Autodesk Inventor part; units mm, degrees
ref_plane "YZ Plane" through (0, 0, 0) normal (1, 0, 0) x (0, 1, 0)
ref_plane "XZ Plane" through (0, 0, 0) normal (0, 1, 0) x (-1, 0, 0)
ref_plane "XY Plane" through (0, 0, 0) normal (0, 0, 1) x (1, 0, 0)
sketch "Sketch1" plane through (0, 0, 0) normal (0, 0, 1) x (1, 0, 0)
  line L0 (0, 0) -> (30, 0)
  line L1 (30, 0) -> (30, 8)
  line L2 (30, 8) -> (0, 8)
  line L3 (0, 8) -> (0, 0)
  line L4 (14.9976, 2) -> (24.9976, 2)
  line L5 (14.9976, 2) -> (4.9976, 2)
  arc A0 (24.9976, 2) -> (4.9976, 2) centre (14.9976, -10.49) ccw
  dimension "d2" = 30
  dimension "d3" = 8
  dimension "d6" = 10
  dimension "d7" = 10
  dimension "d8" = 2
  dimension "d9" = 16
extrude "Extrusion1" add sketch "Sketch1" along normal blind 250
sketch "Sketch2" plane through (0, 8, 0) normal (0, 1, 0) x (1, 0, 0)
  line L0 (30, 0) -> (0, 0)
  line L1 (30, 0) -> (30, -250)
  circle A0 centre (15, -125) radius 5
  line L2 (30, -250) -> (0, -250)
  line L3 (10, -15) -> (10, -5)
  line L4 (10, -5) -> (20, -5)
  line L5 (20, -5) -> (20, -15)
  line L6 (20, -15) -> (10, -15)
  line L7 (10, -15) -> (20, -5) construction
  line L8 (10, -5) -> (20, -15) construction
  line L9 (0, 0) -> (0, -250)
  line L10 (10, -235) -> (10, -245)
  line L11 (10, -245) -> (20, -245)
  line L12 (20, -245) -> (20, -235)
  line L13 (20, -235) -> (10, -235)
  line L14 (10, -235) -> (20, -245) construction
  line L15 (10, -245) -> (20, -235) construction
  point P0 (15, 0)
  point P1 (30, -125)
  point P2 (15, -5)
  point P3 (15, -10)
  point P4 (15, -240)
  point P5 (15, -245)
  dimension "d13" = 10
  dimension "d14" = 120
  dimension "d16" = 0
  dimension "d17" = 125
  dimension "d19" = 5
  dimension "d20" = 10
  dimension "d21" = 10
  dimension "d22" = 5
  dimension "d23" = 10
  dimension "d24" = 5
  dimension "d25" = 5
  dimension "d26" = 10
extrude "Extrusion2" cut sketch "Sketch2" against normal up to surface (8 mm away) from surface at 0 contours A0 | L3 L4 L5 L6 | L13 L12 L11 L10
sketch "Sketch3" plane through (0, 8, 0) normal (0, 1, 0) x (1, 0, 0)
  line L0 (30, 0) -> (30, -250)
  line L1 (30, 0) -> (0, 0)
  line L2 (0, -140) -> (30, -140)
  line L3 (30, -140) -> (30, -110)
  line L4 (30, -110) -> (0, -110)
  line L5 (0, -110) -> (0, -140)
  line L6 (0, -140) -> (30, -110) construction
  line L7 (30, -140) -> (0, -110) construction
  line L8 (4.9976, 0) -> (4.9976, -250)
  point P0 (30, -125)
  point P1 (15, 0)
  point P2 (15, -125)
  dimension "d29" = 15
  dimension "d30" = 125
  dimension "d31" = 30
  dimension "d32" = 30
extrude "Extrusion3" cut sketch "Sketch3" against normal blind 5 contours L0 L2 L8 L4 | L8 L2 L5 L4
properties part number "bridge1"
The model under review builds one solid part; all positions refer to its coordinate system, in mm. A direction names the side the tool comes from. Round coordinates to 2 decimals unless told otherwise and drop trailing zeros. Write each loop counter-clockwise with the first axis right and the second up, starting at its lowest first coordinate (ties: lowest second). Pieces come first, ordered by that corner, then holes. Notation, with made-up numbers: M 43.25,-34.5 L 54.25,-34.5 A22 cw 54.25,-22.5 Z; hole C -34,-27.75 d2. An arc over 180 degrees is marked long. Answer as CSV lines item,"result". Start each with the question number.
Q1. Consider section A-A, the plane z = 94. Give the boundary of the cut face in (x, y), then the cut area to 3 significant figures.
Q2. Consider section C-C, the plane z = 125. Give the boundary of the cut face in (x, y), then the cut area to 3 significant figures.
Q3. Consider section B-B, the plane x = 15. State how many separate pieces and enclosed holes the cut face has, then the cut area to 3 significant figures.
Q4. The part is to be moulded in two halves that separate along X. For faces 1 (the face through (8, 2, 123)), 2 (the face through (0, 2, 123)), 3 (the face through (27, 3, 125)), 4 (the face through (30, 2, 123)), say which applies: +X half, -X half, draft (parallel to the pull), parting line (faces both ways), or undercut.
Q5. Tool access review of faces 5 (the face through (17.307, 1.014, 129.436)), 6 (the face through (15, 6, 140)): name each direction out of +Z, -Z, +X, -X, +Y, -Y from which nothing blocks a thin tool from reaching the whole face with its end or side.
Q6. Wall thickness on line 1 along Z through (x, y) = (15, 1.25); line 2 along Z through (x, y) = (18.5, 7.5); line 3 along X through (y, z) = (0.65, 125): over which ranges is each line inside the solid? List them lowest first.
Result set:
1,outline,"M 0,0 L 30,0 L 30,8 L 0,8 Z; hole M 5,2 L 25,2 A16 ccw Z"
1,area,"192 mm²"
2,outline,"M 0,0 L 10,0 L 10,2 L 5,2 A16 cw 6.39,3 L 0,3 Z; M 20,0 L 30,0 L 30,3 L 23.6,3 A16 cw 25,2 L 20,2 Z"
2,area,"51.3 mm²"
3,separate pieces,"8"
3,enclosed holes,"0"
3,area,"938 mm²"
4,face 1,"undercut"
4,face 2,"-X half"
4,face 3,"draft"
4,face 4,"+X half"
5,face 5,"+Y, -Y"
5,face 6,"+X, -X, +Y"
6,line 1,"z = 0 to 5, 15 to 120, 130 to 235, 245 to 250"
6,line 2,"z = 0 to 5, 15 to 110, 140 to 235, 245 to 250"
6,line 3,"x = 0 to 10, 20 to 30"
